Part model, mm, in its own coordinate system. A direction names the side the tool comes from. Coordinates: 2 decimals unless noted, no trailing zeros. Loops run counter-clockwise (first coordinate to the right, second up) from the corner with the lowest first, then second, coordinate; pieces in that order, holes last.
Autodesk Inventor part; units mm, degrees
ref_plane "YZ Plane" through (0, 0, 0) normal (1, 0, 0) x (0, 1, 0)
ref_plane "XZ Plane" through (0, 0, 0) normal (0, 1, 0) x (-1, 0, 0)
ref_plane "XY Plane" through (0, 0, 0) normal (0, 0, 1) x (1, 0, 0)
sketch "スケッチ1" plane through (0, 0, 0) normal (0, 1, 0) x (-1, 0, 0)
  line L0 (-47, -9.5) -> (47, -9.5)
  line L1 (47, -9.5) -> (47, 9.5)
  line L2 (47, 9.5) -> (-47, 9.5)
  line L3 (-47, 9.5) -> (-47, -9.5)
  line L4 (-47, -9.5) -> (47, 9.5) construction
  line L5 (47, -9.5) -> (-47, 9.5) construction
  point P0 (0, 0)
  dimension "d0" = 94
  dimension "d1" = 19
extrude "プレート1" add sketch "スケッチ1" along normal blind 2
sketch "スケッチ2" plane through (45, 0, -9.5) normal (1, 0, 0) x (0, 1, 0)
  line L0 (0, 19) -> (0, 0)
  line L1 (0, 0) -> (25, 0)
  line L2 (25, 0) -> (25, 19)
  line L3 (25, 19) -> (0, 19)
edge flange "フランジ1" height 25 angle 90 thickness 2 bend radius 2 thickness toward (1, 0, 0) relief tear relief width 2 relief depth 1 edges at (47, 2, 0) wall of the first edge with corners at (45, 0, 9.5) (45, 0, -9.5) (45, 25, -9.5) (45, 25, 9.5)
bend "曲げ1"
corner "コーナー1"
sketch "スケッチ3" plane through (-45, 0, 9.5) normal (-1, 0, 0) x (0, -1, 0)
  line L0 (0, -19) -> (0, 0)
  line L1 (0, 0) -> (-25, 0)
  line L2 (-25, 0) -> (-25, -19)
  line L3 (-25, -19) -> (0, -19)
edge flange "フランジ2" height 25 angle 90 thickness 2 bend radius 2 thickness toward (-1, 0, 0) relief tear relief width 2 relief depth 1 edges at (-47, 2, 0) wall of the first edge with corners at (-45, 0, -9.5) (-45, 0, 9.5) (-45, 25, 9.5) (-45, 25, -9.5)
bend "曲げ2"
corner "コーナー2"
sketch "スケッチ5" plane through (0, 0, 0) normal (0, -1, 0) x (1, 0, 0)
  arc A0 (-35, 2) -> (-35, -2) centre (-35, 0) ccw
  arc A1 (35, -2) -> (35, 2) centre (35, 0) ccw
  line L0 (-35, 2) -> (35, 2)
  line L1 (35, -2) -> (-35, -2)
  point P0 (0, 0)
  dimension "d31" = 4
  dimension "d32" = 2
  dimension "d33" = 2
  dimension "d34" = 2
  dimension "d35" = 35
  dimension "d36" = 35
extrude "押し出し1" cut sketch "スケッチ5" against normal blind 2
sketch "スケッチ6" plane through (47, 25, 9.5) normal (1, 0, 0) x (0, 0, -1)
  point P0 (9.5, -25)
sketch "スケッチ7" plane through (47, 25, 9.5) normal (1, 0, 0) x (0, 0, -1)
  line L0 (7.5, -4) -> (7.5, -17)
  arc A0 (7.5, -17) -> (11.5, -17) centre (9.5, -17) ccw
  line L1 (11.5, -17) -> (11.5, -4)
  arc A1 (11.5, -4) -> (7.5, -4) centre (9.5, -4) ccw
  line L2 (0, 0) -> (19, 0)
  line L3 (0, -21) -> (19, -21)
  point P0 (9.5, -25)
  point P1 (9.5, 0)
  dimension "d45" = 4
  dimension "d46" = 4
  dimension "d47" = 2
extrude "押し出し2" cut sketch "スケッチ7" against normal blind 100
equation "\"d2\" = Thickness"
equation "\"d3\" = BendReliefWidth"
equation "\"d4\" = BendReliefDepth"
equation "\"d5\" = MinimumRemnant"
equation "\"d6\" = TransitionRadius"
equation "\"d9\" = BendRadius"
equation "\"d10\" = CornerReliefSize"
equation "\"d11\" = GapSize"
equation "\"d12\" = JacobiRadiusSize"
equation "\"d13\" = BendReliefWidth"
equation "\"d14\" = BendReliefDepth"
equation "\"d15\" = MinimumRemnant"
equation "\"d16\" = TransitionRadius"
equation "\"d19\" = BendRadius"
equation "\"d20\" = CornerReliefSize"
equation "\"d21\" = GapSize"
equation "\"d22\" = JacobiRadiusSize"
equation "\"BendRadius\" = Thickness"
equation "\"BendReliefWidth\" = Thickness"
equation "\"BendReliefDepth\" = 0.5 * Thickness"
equation "\"CornerReliefSize\" = 4 * Thickness"
equation "\"MinimumRemnant\" = 2 * Thickness"
equation "\"TransitionRadius\" = BendRadius"
equation "\"JacobiRadiusSize\" = BendRadius"
equation "\"GapSize\" = Thickness"
properties part number "cup" material "アルミニウム 6061"
Q1. Saw through at C-C (x = -4). List the corners of the cut face in (y, z), plus the area to 3 significant figures.
Q2. Mould opens along Z. For faces 1 (the cylindrical face through (-44.43, 2.6, 0.13)), 2 (the flat face through (0, 1, 9.5)), 3 (the cylindrical face through (46, 6, 0)) say: released by +Z, released by -Z, zero draft, split by the parting line, or undercut.
Q3. Saw through at B-B (z = 0). List the corners of the cut face in (x, y).
Q4. Tool access for faces 4 (the cylindrical face through (44.43, 2.6, -0.13)), 5 (the flat face through (-47, 14.6, 2.2)), 6 (the flat face through (0, 1, -2)), 7 (the flat face through (46, 25, 0)), 8 (the flat face through (46, 15, 2)): list every direction of +Z, -Z, +X, -X, +Y, -Y with a clear straight run to the whole face (end or side of a thin tool).
Q5. Saw through at A-A (y = 9). List the corners of the cut face in (x, z).
Q6. Probe line 1 (X direction, y = 17, z = 8.5); line 2 (Y direction, x = -10.5, z = -5.75). List the from-to ranges inside material, lowest first.
Q7. Drop a flat-ended pin along its axis: P1, Ø3, axis at x = -32, z = -5, coming from the +Y side. Give the stop position or say it passes through.
Q8. Saw through at D-D (z = 3.5). List the corners of the cut face in (x, y), plus the area to 3 significant figures.
Checked values:
1. outline: (0, -9.5) - (2, -9.5) - (2, -2) - (0, -2) - close; (0, 2) - (2, 2) - (2, 9.5) - (0, 9.5) - close
1. area: 30.0 mm2
2. face 1: zero draft
2. face 2: released by +Z
2. face 3: undercut
3. outline: (-47, 4) arc R4 ccw to (-43, 0) - (-37, 0) - (-37, 2) - (-43, 2) arc R2 cw to (-45, 4) - (-45, 6) - (-47, 6) - close; (-47, 23) - (-45, 23) - (-45, 25) - (-47, 25) - close; (37, 0) - (43, 0) arc R4 ccw to (47, 4) - (47, 6) - (45, 6) - (45, 4) arc R2 cw to (43, 2) - (37, 2) - close; (45, 23) - (47, 23) - (47, 25) - (45, 25) - close
4. face 4: +Z, -Z, +Y
4. face 5: +Z, -Z, -X, +Y, -Y
4. face 6: +Y, -Y
4. face 7: +Z, -Z, +X, -X, +Y
4. face 8: +X, -X
5. outline: (-47, -9.5) - (-45, -9.5) - (-45, -2) - (-47, -2) - close; (-47, 2) - (-45, 2) - (-45, 9.5) - (-47, 9.5) - close; (45, -9.5) - (47, -9.5) - (47, -2) - (45, -2) - close; (45, 2) - (47, 2) - (47, 9.5) - (45, 9.5) - close
6. line 1: x = -47 to -45, 45 to 47
6. line 2: y = 0 to 2
7. P1: stops at y = 2
8. outline: (-47, 4) arc R4 ccw to (-43, 0) - (43, 0) arc R4 ccw to (47, 4) - (47, 25) - (45, 25) - (45, 4) arc R2 cw to (43, 2) - (-43, 2) arc R2 cw to (-45, 4) - (-45, 25) - (-47, 25) - close
8. area: 275 mm2
